Here's how the part is built. I have some questions about the finished solid (model axes, mm). A direction names the side the tool comes from. Give positions to 0.01 mm unless a question says otherwise; leave off trailing zeros. Loops run counter-clockwise (first coordinate to the right, second up) from the corner with the lowest first, then second, coordinate; pieces in that order, holes last. Notation, with made-up numbers: (27, -7) - (51, -7) arc R21 cw to (51, -3) - close; hole circle Ø5 at (-18.75, -22). An arc over 180 degrees is marked (long way). Use a Markdown table: item, result.
Autodesk Inventor part; units mm, degrees
ref_plane "YZ Plane" through (0, 0, 0) normal (1, 0, 0) x (0, 1, 0)
ref_plane "XZ Plane" through (0, 0, 0) normal (0, 1, 0) x (-1, 0, 0)
ref_plane "XY Plane" through (0, 0, 0) normal (0, 0, 1) x (1, 0, 0)
sketch "Skizze1" plane through (0, 0, 0) normal (0, 1, 0) x (-1, 0, 0)
  circle A0 centre (0, 0) radius 3.4
  dimension "d0" = 6.8
extrude "Extrusion1" add sketch "Skizze1" along normal blind 10
sketch "Skizze2" plane through (0, 10, 0) normal (0, 1, 0) x (1, 0, 0)
  line L0 (-3.1754, 0) -> (-1.5877, 2.75)
  line L1 (-1.5877, 2.75) -> (1.5877, 2.75)
  line L2 (1.5877, 2.75) -> (3.1754, 0)
  line L3 (3.1754, 0) -> (1.5877, -2.75)
  line L4 (1.5877, -2.75) -> (-1.5877, -2.75)
  line L5 (-1.5877, -2.75) -> (-3.1754, 0)
  line L6 (3.1754, 0) -> (-3.1754, 0) construction
  line L7 (-4.76, 0) -> (4.76, 0) construction
  point P0 (0, 0)
  point P1 (0, 0)
  dimension "d10" = 5.5
extrude "Extrusion2" cut sketch "Skizze2" against normal blind 2.4
hole "Bohrung2" at (0, 0, 0) direction (0, 1, 0) diameter 3.4 end through all
sketch "Skizze3" plane through (0, 0, 0) normal (1, 0, 0) x (0, 1, 0)
  circle A0 centre (5, 3.1) radius 0.5
  line L0 (10, 2.75) -> (10, 0)
  line L1 (0, 0) -> (10, 0) construction
  circle A1 centre (2, 3.1) radius 0.5
  line L2 (2, 3.1) -> (5, 3.1) construction
  line L3 (0, 3.4) -> (10, 3.4)
  point P0 (1.6, 3.4)
  point P1 (2.4, 3.4)
  point P2 (4.6, 3.4)
  point P3 (5.4, 3.4)
  dimension "d21" = 3.1
  dimension "d22" = 5
  dimension "d23" = 3
  dimension "d24" = 1
revolve "Umdrehung1" add sketch "Skizze3" angle 360 about axis through (0, 0, 0) along (0, 1, 0) picked at (1.8932, 3.428) picked at (4.8932, 3.428) contours L3 A1 | L3 A0
properties part number "Tuebel"
(1) We'd pull the mould along X, two halves only. Please class faces 1 (the face through (0, 10, -3)), 2 (the face through (0, 9, -2.75)), 3 (the face through (0.74, 0.79, 3.32)): pulls with the +X half, pulls with the -X half, needs draft (parallel to the pull), parting line crosses it, or undercut.
A:
| item | result |
|---|---|
| face 1 | needs draft |
| face 2 | undercut |
| face 3 | parting line crosses it |
(2) Suppose I cut it at B-B on y = 8. Write out the boundary of the cut face in (x, z), plus the area to 3 significant figures.
A:
| item | result |
|---|---|
| outline | circle Ø6.8 at (0, 0); hole (-3.18, 0) - (-1.59, -2.75) - (1.59, -2.75) - (3.18, 0) - (1.59, 2.75) - (-1.59, 2.75) - close |
| area | 10.1 mm2 |
(3) On a 3-axis mill with a long thin cutter (end or side, diameter ignored), from which of +Z, -Z, +X, -X, +Y, -Y can I reach the whole of each face in a straight line? I mean faces 4 (the face through (0.74, 3.48, 3.32)), 5 (the face through (0, 9, 2.75)), 6 (the face through (1.66, 3.85, 0.37)). Say none if no direction works.
A:
| item | result |
|---|---|
| face 4 | none |
| face 5 | +Y |
| face 6 | +Y, -Y |
(4) Suppose I cut it at A-A on x = 0. Write out the boundary of the cut face in (y, z), plus the area to 3 significant figures.
A:
| item | result |
|---|---|
| outline | (0, -3.4) - (1.6, -3.4) arc R0.5 ccw to (2.4, -3.4) - (4.6, -3.4) arc R0.5 ccw to (5.4, -3.4) - (10, -3.4) - (10, -2.75) - (7.6, -2.75) - (7.6, -1.7) - (0, -1.7) - close; (0, 1.7) - (7.6, 1.7) - (7.6, 2.75) - (10, 2.75) - (10, 3.4) - (5.4, 3.4) arc R0.5 ccw to (4.6, 3.4) - (2.4, 3.4) arc R0.5 ccw to (1.6, 3.4) - (0, 3.4) - close |
| area | 29.4 mm2 |
(5) Will these pins go through, and if not, where does the flat tip stop? pin 1 (1 mm diameter, centred on y = 5.5, z = -2, fed in from -X); pin 2 (2.5 mm diameter, centred on x = -0.5, y = 8.5, fed in from -Z); pin 3 (1.9 mm diameter, centred on x = -0.5, y = 8.5, fed in from +Z).
A:
| item | result |
|---|---|
| pin 1 | x = -3.18 |
| pin 2 | z = -3.4 |
| pin 3 | z = 3.4 |
(6) If I drill on line 1 (X direction, y = 3.5, z = 0); line 2 (X direction, y = 2.75, z = 1.5), over which ranges is the centre line in solid material (lowest first)?
A:
| item | result |
|---|---|
| line 1 | -3.4 to -1.7, 1.7 to 3.4 |
| line 2 | -3.05 to -0.8, 0.8 to 3.05 |
(7) Suppose I cut it at C-C on y = 4. Write out the boundary of the cut face in (x, z).
A:
| item | result |
|---|---|
| outline | circle Ø6.8 at (0, 0); hole circle Ø3.4 at (0, 0) |
